from build123d import *

# Parameters (mm, degrees)
F1_DEPTH = 57.15
F2_R     = 5.08


with BuildPart() as f1:
    # F0 (on Front) → F1 (new body)
    with BuildSketch(Plane.XZ):
        with BuildLine():
            Line((144.78, 324.792413), (157.48, 346.9309))
            ThreePointArc((157.48, 346.9309), (0, 381), (-157.48, 346.9309))
            Line((-157.48, 346.9309), (-144.78, 324.792413))
            ThreePointArc((-144.78, 324.792413), (0, 355.6), (144.78, 324.792413))
        make_face()
    extrude(amount=-F1_DEPTH)

    # F2
    f2_edges = [f1.edges().sort_by_distance(p)[0] for p in [
        (0, 0, 355.6),
        (0, 0, 381),
        (0, 57.15, 381),
        (0, 57.15, 355.6),
    ]]
    fillet(f2_edges, radius=F2_R)


solid = f1.part
Can you work these out from the model? Positions are in its coordinate system, mm. Give positions to 0.01 mm unless a question says otherwise; leave off trailing zeros. Loops run counter-clockwise (first coordinate to the right, second up) from the corner with the lowest first, then second, coordinate; pieces in that order, holes last. Notation, with made-up numbers: (-30.5, 84.5) - (-15.5, 84.5) arc R18 cw to (-15.5, 93.5) - close; hole circle Ø10 at (13, 7.25). An arc over 180 degrees is marked (long way). One line per item, written item: value.
(1) I'm going to push flat-ended pins straight in: pin 1 (10 mm diameter, centred on x = 48.5, y = 50.5, fed in from -Z); pin 2 (8 mm diameter, centred on x = -116, z = 333.5, fed in from -Y); pin 3 (1 mm diameter, centred on x = 50, z = 355.5, fed in from -Y). Where does each tip first touch, or does it pass through?
Verdict:
pin 1: z = 351.55
pin 2: y = 1.48
pin 3: y = 0.14
(2) If we section it at A-A, the plane y = 46: List the corners of the cut face in (x, z) for me, plus the area to 3 significant figures.
Verdict:
outline: (-157.48, 346.93) - (-144.78, 324.79) arc R355.6 cw to (144.78, 324.79) - (157.48, 346.93) arc R381 ccw to start
area: 7,910 mm^2
(3) I need wall thicknesses on line 1 along Z through (x, y) = (5, 8.5); line 2 along Z through (x, y) = (91, 11); line 3 along Y through (x, z) = (136, 355.5). Which ranges of each line are inside material? Lowest first, please.
Verdict:
line 1: 355.56 to 380.97
line 2: 343.76 to 369.97
line 3: 3.17 to 53.98
(4) If we mould it in two halves opening along X, with no side actions, what happens to faces 1 (the face through (-151.22, 28.17, 336.02)), 2 (the face through (2.273, 28.246, 380.993)), 3 (the face through (-2.088, 28.246, 355.594)), 4 (the face through (-1, 0, 361))? For each: released by +X, released by -X, zero draft, split by the parting line, or undercut.
Verdict:
face 1: released by -X
face 2: split by the parting line
face 3: undercut
face 4: zero draft
